Source: CAD feature listing. Evaluate the final solid. Frame: model axes, mm. A direction names the side the tool comes from. Give positions to 0.01 mm unless a question says otherwise; leave off trailing zeros. Order: outer loops, then holes, each group sorted by start corner. A loop starts at its lowest first (then second) coordinate and runs counter-clockwise, first axis right, second up.
```python
from build123d import *

# Parameters (mm, degrees)
IMPORTED_START                     = -42
IMPORTED_BODY_1_OUTLINE_R          = 1.75
IMPORTED_BODY_1_DEPTH              = 2
EXTRUDE_START                      = -2.01012
SKETCH_1_R                         = 1.75
EXTRUDE_1_DEPTH                    = 2.01012
SKETCH_2_R                         = 2.5
SKETCH_2_R_2                       = 0.85
EXTRUDE_2_DEPTH                    = 5
FILLET_1_R                         = 1
CHAMFER_1_SIZE                     = 0.6
SKETCH_3_R                         = 0.85
CUT_EXTRUDE_1_DEPTH                = 83.477440833
PATTERN_LINEAR_1_COUNT             = 2
PATTERN_LINEAR_1_PITCH             = 58
PATTERN_LINEAR_1_COUNT_DIR2        = 2
PATTERN_LINEAR_1_PITCH_DIR2        = 23
FILLET_1_OF_PATTERN_LINEAR_1_R     = 1
CHAMFER_1_OF_PATTERN_LINEAR_1_SIZE = 0.6


# Read off the part's stored shape, not the designer's step: Заготовка-Основание-1
with BuildPart() as part:
    # Заготовка-Основание-1 outline → Заготовка-Основание-1 (new body)
    with BuildSketch(Plane.XY.offset(IMPORTED_START)):
        with BuildLine():
            add(Edge.make_bspline(
                [(-52.567338158, -56.687092755), (-53.907083637, -52.949373723), (-55.113256729, -49.167125614), (-56.183975236, -45.347636311)],
                knots=[0.154838503, 0.154838503, 0.154838503, 0.154838503, 0.226015104, 0.226015104, 0.226015104, 0.226015104], degree=3))
            ThreePointArc((-52.567338158, -56.687092755), (-50.738457524, -59.088732308), (-47.860564525, -60))
            Line((-47.860564525, -60), (-41.924542191, -60))
            ThreePointArc((-41.924542191, -60), (-39.685256286, -59.470525543), (-37.920228255, -57.994239454))
            ThreePointArc((-37.920228255, -57.994239454), (0, -39), (37.920228255, -57.994239454))
            ThreePointArc((37.920228255, -57.994239454), (39.685256286, -59.470525543), (41.924542191, -60))
            Line((41.924542191, -60), (47.860564525, -60))
            ThreePointArc((47.860564525, -60), (50.738457524, -59.088732308), (52.567338158, -56.687092755))
            add(Edge.make_bspline(
                [(56.183975236, -45.347636311), (55.113256729, -49.167125614), (53.907083637, -52.949373723), (52.567338158, -56.687092755)],
                knots=[0.773984896, 0.773984896, 0.773984896, 0.773984896, 0.845161497, 0.845161497, 0.845161497, 0.845161497], degree=3))
            ThreePointArc((56.183975236, -45.347636311), (56.122806116, -42.446648473), (54.460846844, -40.068127194))
            ThreePointArc((54.460846844, -40.068127194), (35, 6e-09), (54.460846854, 40.068127202))
            ThreePointArc((54.460846854, 40.068127202), (56.122806127, 42.446648481), (56.183975247, 45.34763632))
            add(Edge.make_bspline(
                [(52.567338167, 56.687092757), (53.907083647, 52.949373727), (55.113256739, 49.167125621), (56.183975247, 45.34763632)],
                knots=[0.15483858, 0.15483858, 0.15483858, 0.15483858, 0.226015181, 0.226015181, 0.226015181, 0.226015181], degree=3))
            ThreePointArc((52.567338167, 56.687092757), (50.738457533, 59.088732309), (47.860564535, 60))
            Line((47.860564535, 60), (-47.860564535, 60))
            ThreePointArc((-47.860564535, 60), (-50.738457533, 59.088732309), (-52.567338167, 56.687092757))
            add(Edge.make_bspline(
                [(-56.183975247, 45.34763632), (-55.113256739, 49.167125621), (-53.907083647, 52.949373727), (-52.567338167, 56.687092757)],
                knots=[0.773984819, 0.773984819, 0.773984819, 0.773984819, 0.84516142, 0.84516142, 0.84516142, 0.84516142], degree=3))
            ThreePointArc((-56.183975247, 45.34763632), (-56.122806127, 42.446648481), (-54.460846854, 40.068127202))
            ThreePointArc((-54.460846854, 40.068127202), (-35, 6e-09), (-54.460846844, -40.068127194))
            ThreePointArc((-54.460846844, -40.068127194), (-56.122806116, -42.446648473), (-56.183975236, -45.347636311))
        make_face()
        with Locations((-48.510868396, -50)):
            Circle(IMPORTED_BODY_1_OUTLINE_R, mode=Mode.SUBTRACT)
        with Locations((-25, -29)):
            Circle(IMPORTED_BODY_1_OUTLINE_R, mode=Mode.SUBTRACT)
        with Locations((48.510868396, -50)):
            Circle(IMPORTED_BODY_1_OUTLINE_R, mode=Mode.SUBTRACT)
        with Locations((25, -29)):
            Circle(IMPORTED_BODY_1_OUTLINE_R, mode=Mode.SUBTRACT)
        with Locations((-48.510868396, 50)):
            Circle(IMPORTED_BODY_1_OUTLINE_R, mode=Mode.SUBTRACT)
        with Locations((-25, 50)):
            Circle(IMPORTED_BODY_1_OUTLINE_R, mode=Mode.SUBTRACT)
        with BuildLine():
            Line((-15, -14), (-15, 35))
            ThreePointArc((-15, 35), (-13.535533906, 38.535533906), (-10, 40))
            Line((-10, 40), (10, 40))
            ThreePointArc((10, 40), (13.535533906, 38.535533906), (15, 35))
            Line((15, 35), (15, -14))
            ThreePointArc((15, -14), (13.535533906, -17.535533906), (10, -19))
            Line((10, -19), (-10, -19))
            ThreePointArc((-10, -19), (-13.535533906, -17.535533906), (-15, -14))
        make_face(mode=Mode.SUBTRACT)
        with Locations((25, 50)):
            Circle(IMPORTED_BODY_1_OUTLINE_R, mode=Mode.SUBTRACT)
        with Locations((48.510868396, 50)):
            Circle(IMPORTED_BODY_1_OUTLINE_R, mode=Mode.SUBTRACT)
    extrude(amount=IMPORTED_BODY_1_DEPTH)

    # Эскиз1 → Бобышка-Вытянуть1 (add)
    with BuildSketch(Plane(origin=(0, 0, -42), x_dir=(-1, 0, 0), z_dir=(0, 0, -1)).offset(EXTRUDE_START)):
        with Locations((-25, -29)):
            Circle(SKETCH_1_R)
        with Locations((25, -29)):
            Circle(SKETCH_1_R)
        with Locations((25, 50)):
            Circle(SKETCH_1_R)
        with Locations((-25, 50)):
            Circle(SKETCH_1_R)
        with BuildLine():
            Line((-10, -19), (10, -19))
            ThreePointArc((10, -19), (13.535533906, -17.535533906), (15, -14))
            Line((15, -14), (15, 35))
            ThreePointArc((15, 35), (13.535533906, 38.535533906), (10, 40))
            Line((10, 40), (-10, 40))
            ThreePointArc((-10, 40), (-13.535533906, 38.535533906), (-15, 35))
            Line((-15, 35), (-15, -14))
            ThreePointArc((-15, -14), (-13.535533906, -17.535533906), (-10, -19))
        make_face()
    extrude(amount=EXTRUDE_1_DEPTH)

    # Эскиз2 → Бобышка-Вытянуть2 (add)
    with BuildSketch(Plane(origin=(0, 0, -42), x_dir=(-1, 0, 0), z_dir=(0, 0, -1))):
        with Locations((-11.5, 29)):
            Circle(SKETCH_2_R)
        with Locations((-11.5, 29)):
            Circle(SKETCH_2_R_2, mode=Mode.SUBTRACT)
    extrude_2 = extrude(amount=EXTRUDE_2_DEPTH)

    # Скругление1
    fillet_1_edges = [part.edges().sort_by_distance(p)[0] for p in [
        (14, 29, -42),
    ]]
    fillet(fillet_1_edges, radius=FILLET_1_R)

    # Фаска1
    chamfer_1_edges = [part.edges().sort_by_distance(p)[0] for p in [
        (12.35, 29, -47),
    ]]
    chamfer(chamfer_1_edges, length=CHAMFER_1_SIZE)

    # Эскиз3 → Вырез-Вытянуть1 (cut, through all)
    with BuildSketch(Plane(origin=(0, 0, -42), x_dir=(-1, 0, 0), z_dir=(0, 0, -1))):
        with Locations((-11.5, 29)):
            Circle(SKETCH_3_R)
    cut_extrude_1 = extrude(amount=-CUT_EXTRUDE_1_DEPTH, mode=Mode.SUBTRACT)

    # Линейный массив1: Бобышка-Вытянуть2, Cut-Extrude 1 2 × 2
    with Locations(*[(-j * PATTERN_LINEAR_1_PITCH_DIR2, -i * PATTERN_LINEAR_1_PITCH, 0) for i in range(PATTERN_LINEAR_1_COUNT) for j in range(PATTERN_LINEAR_1_COUNT_DIR2) if (i, j) != (0, 0)]):
        add(extrude_2)
        add(cut_extrude_1, mode=Mode.SUBTRACT)

    # Скругление1 of Линейный массив1
    fillet_1_of_pattern_linear_1_edges = [part.edges().sort_by_distance(p)[0] for p in [
        (-9, 29, -42),
        (14, -29, -42),
        (-9, -29, -42),
    ]]
    fillet(fillet_1_of_pattern_linear_1_edges, radius=FILLET_1_OF_PATTERN_LINEAR_1_R)

    # Фаска1 of Линейный массив1
    chamfer_1_of_pattern_linear_1_edges = [part.edges().sort_by_distance(p)[0] for p in [
        (-10.65, 29, -47),
        (12.35, -29, -47),
        (-10.65, -29, -47),
    ]]
    chamfer(chamfer_1_of_pattern_linear_1_edges, length=CHAMFER_1_OF_PATTERN_LINEAR_1_SIZE)


solid = part.part
```
1) Draft query along X for faces 3 (the cylindrical face through (-11.17, -26.52, -44.97)), 4 (the flat face through (-13, -30, -47)), 5 (the cylindrical face through (35.004, -0.645, -41.014)). Return one class per face: +X half, -X half, draft (parallel to the pull), parting line (faces both ways), or undercut.
Report:
face 3: undercut
face 4: draft
face 5: +X half
2) Section query A-A, the plane x = -36.5. Return the cut outline in (y, z), and give its area (3 significant figures).
Report:
outline: (-56.19, -42) - (-12.28, -42) - (-12.28, -40) - (-56.19, -40) - close; (12.28, -42) - (60, -42) - (60, -40) - (12.28, -40) - close
area: 183 mm2
3) Section query D-D, the plane x = 40. Return the cut outline in (y, z), and give its area (3 significant figures).
Report:
outline: (-59.61, -42) - (-22.02, -42) - (-22.02, -40) - (-59.61, -40) - close; (22.02, -42) - (60, -42) - (60, -40) - (22.02, -40) - close
area: 151 mm2
4) Material intervals for L1, parallel to X at y = -29.5, z = -46.5; L2, parallel to Z at x = -20, y = -4; L3, parallel to Y at x = -51, z = -41.25, sorted ascending.
Report:
L1: x = -13.95 to -12.31, -10.69 to -9.05, 9.05 to 10.69, 12.31 to 13.95
L2: z = -42 to -40
L3: y = -58.89 to -37.09, 37.09 to 58.89
5) Reachability of faces 1 (the flat face through (-25, -29, -39.99)), 2 (the cylindrical face through (11.83, 31.48, -44.97)) from +Z, -Z, +X, -X, +Y, -Y: full face, straight path, thin tool, end or side. Return the list, or none.
Report:
face 1: +Z, +X, -X, +Y, -Y
face 2: -Z
6) Pin query (flat end, axial travel): pin 1 (2.5 mm diameter, centred on x = -11.5, y = -29, fed in from +Z); pin 2 (1 mm diameter, centred on x = -6, y = 47, fed in from -Z); pin 3 (4 mm diameter, centred on y = -9.5, z = -42, fed in from +X). Return the tip coordinate at first contact, or that it passes through.
Report:
pin 1: stops at z = -40
pin 2: stops at z = -42
pin 3: stops at x = 36.31
